The listing builds one solid part. Answer for the finished solid, in the listing's coordinates (mm). Face numbers are marked on the shaded views. A direction names the side the tool comes from. Give positions to 0.01 mm unless a question says otherwise; leave off trailing zeros. Order: outer loops, then holes, each group sorted by start corner. A loop starts at its lowest first (then second) coordinate and runs counter-clockwise, first axis right, second up.
```python
from build123d import *

# Parameters (mm, degrees)
F1_DEPTH = 20
F2_W     = 20
F2_H     = 20
F3_DEPTH = 26.001
F5_DEPTH = 40.001


with BuildPart() as f1:
    # F0 (on Top) → F1 (new body, symmetric)
    with BuildSketch(Plane.XY):
        Polygon((0, 26), (0, 0), (10, 0), (10, 13), (50, 13), (50, 39), (40, 39), (40, 26), align=None)
    extrude(amount=F1_DEPTH, both=True)

    # F2 (on face) → F3 (cut, through all)
    with BuildSketch(Plane.XZ.offset(-13)):
        with Locations((40, 0)):
            Rectangle(F2_W, F2_H)
    extrude(amount=-F3_DEPTH, mode=Mode.SUBTRACT)

    # F4 (on face) → F5 (cut, through all)
    with BuildSketch(Plane.XY.offset(20)):
        Polygon((0, 0), (10, 0), (0, 13), align=None)
    extrude(amount=-F5_DEPTH, mode=Mode.SUBTRACT)


solid = f1.part
```
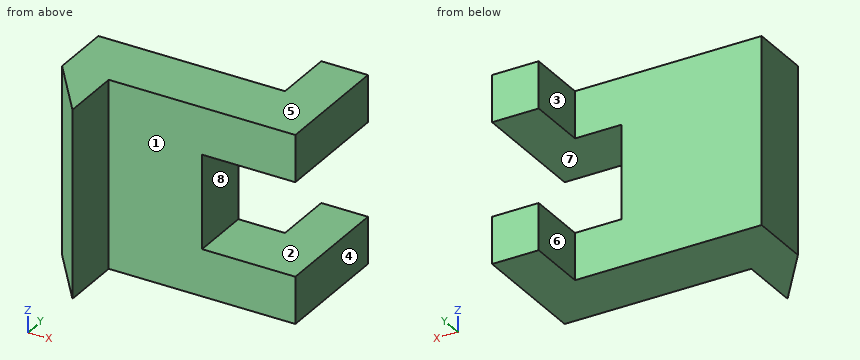
1) A tool of negligible diameter and unlimited length cuts with its end or side. For the marked faces 1, 2, 3 and 4, from which of +Z, -Z, +X, -X, +Y, -Y can it reach the whole face along a straight path? Write none if from no direction.
Geometry says:
face 1: +Z, -Z, +X, -Y
face 2: +X, +Y, -Y
face 3: +Z, -Z, -X, +Y
face 4: +Z, -Z, +X, +Y, -Y
2) Find section D-D (y = 25). Write down the section's boundary in (x, z).
Geometry says:
outline: (0, -20) - (50, -20) - (50, -10) - (30, -10) - (30, 10) - (50, 10) - (50, 20) - (0, 20) - close
3) Given P1, Ø14.5, axis at y = 22, z = -0.5, coming from the +X side; P2, Ø12, axis at x = 12, z = 5.5, coming from the +Y side; P3, Ø5, axis at y = 30, z = -15, coming from the -X side; P4, Ø10, axis at x = 38, z = 2, coming from the +Y side (3 decimals), each flat-ended and moving along its own axis, determine where each tip first touches the part or whether it passes through.
Geometry says:
P1: stops at x = 30
P2: stops at y = 26
P3: stops at x = 40
P4: passes through
4) Find section A-A (x = 42). Write down the section's boundary in (y, z).
Geometry says:
outline: (13, -20) - (39, -20) - (39, -10) - (13, -10) - close; (13, 10) - (39, 10) - (39, 20) - (13, 20) - close
5) Straight lines are drawn through the part: probe 1 along Z at (x, y) = (35.5, 24); probe 2 along Y at (x, z) = (25.5, 12); probe 3 along X at (y, z) = (25.5, -9). For each, find the intervals that lie inside material, in ascending order.
Geometry says:
probe 1: z = -20 to -10, 10 to 20
probe 2: y = 13 to 26
probe 3: x = 0 to 30
6) Find section C-C (y = 29.5). Write down the section's boundary in (x, z).
Geometry says:
outline: (40, -20) - (50, -20) - (50, -10) - (40, -10) - close; (40, 10) - (50, 10) - (50, 20) - (40, 20) - close
7) Find section B-B (z = 17). Write down the section's boundary in (x, y).
Geometry says:
outline: (0, 13) - (10, 0) - (10, 13) - (50, 13) - (50, 39) - (40, 39) - (40, 26) - (0, 26) - close
8) For a pull along Z with two mould halves and no side action, classify the marked faces 5, 6, 7 and 8 as +Z half, -Z half, draft (parallel to the pull), parting line (faces both ways), or undercut.
Geometry says:
face 5: +Z half
face 6: draft
face 7: undercut
face 8: undercut
